The listing builds one solid part. Answer for the finished solid, in the listing's coordinates (mm). A direction names the side the tool comes from. Coordinates: 2 decimals unless noted, no trailing zeros. Order: outer loops, then holes, each group sorted by start corner. A loop starts at its lowest first (then second) coordinate and runs counter-clockwise, first axis right, second up.
```python
from build123d import *

# Parameters (mm, degrees)
SKETCH1_W           = 20
SKETCH1_H           = 18
BOSS_EXTRUDE1_DEPTH = 13
SKETCH7_W           = 3.5
SKETCH7_H           = 5.75
CUT_EXTRUDE6_DEPTH  = 25.351591324
SKETCH2_W           = 5.1
SKETCH2_H           = 11.1
CUT_EXTRUDE1_DEPTH  = 13.75
SKETCH3_R           = 1.05
CUT_EXTRUDE2_DEPTH  = 21.953818268
SKETCH4_R           = 2
CUT_EXTRUDE3_DEPTH  = 1.9
SKETCH11_R          = 0.9
CUT_EXTRUDE9_DEPTH  = 3
SKETCH5_W           = 11.1
SKETCH5_H           = 5.1
CUT_EXTRUDE4_DEPTH  = 19.708286934
SKETCH8_W           = 5.35
SKETCH8_H           = 5.1
SKETCH8_R           = 1.1
BOSS_EXTRUDE2_DEPTH = 1.5
SKETCH10_R          = 0.95
CUT_EXTRUDE8_DEPTH  = 6
SKETCH14_R          = 1.1
CUT_EXTRUDE11_DEPTH = 19.708286934
FILLET2_R           = 1.75
CHAMFER1_SIZE       = 0.5


with BuildPart() as part:
    # Sketch1 → Boss-Extrude1 (new body)
    with BuildSketch(Plane(origin=(0, 0, 0), x_dir=(1, 0, 0), z_dir=(0, 1, 0))):
        Rectangle(SKETCH1_W, SKETCH1_H)
    extrude(amount=BOSS_EXTRUDE1_DEPTH)

    # Sketch7 → Cut-Extrude6 (cut, through all)
    with BuildSketch(Plane.XY.offset(9)):
        with Locations((1, 10.125)):
            Rectangle(SKETCH7_W, SKETCH7_H)
    extrude(amount=-CUT_EXTRUDE6_DEPTH, mode=Mode.SUBTRACT)

    # Sketch2 → Cut-Extrude1 (cut)
    with BuildSketch(Plane.ZY.offset(10)):
        with Locations((-1.45, 7.45)):
            Rectangle(SKETCH2_W, SKETCH2_H)
    extrude(amount=-CUT_EXTRUDE1_DEPTH, mode=Mode.SUBTRACT)

    # Sketch3 → Cut-Extrude2 (cut, through all)
    with BuildSketch(Plane.ZY.offset(-3.75)):
        with Locations((-1.45, 3.9)):
            Circle(SKETCH3_R)
    extrude(amount=-CUT_EXTRUDE2_DEPTH, mode=Mode.SUBTRACT)

    # Sketch4 → Cut-Extrude3 (cut)
    with BuildSketch(Plane(origin=(10, 0, 0), x_dir=(0, 0, -1), z_dir=(1, 0, 0))):
        with Locations((1.45, 3.9)):
            Circle(SKETCH4_R)
    extrude(amount=-CUT_EXTRUDE3_DEPTH, mode=Mode.SUBTRACT)

    # Sketch11 → Cut-Extrude9 (cut)
    with BuildSketch(Plane(origin=(10, 0, 0), x_dir=(0, 0, -1), z_dir=(1, 0, 0))):
        with Locations((4.95, 3.9)):
            Circle(SKETCH11_R)
        with Locations(Location((-2.05, 3.9, 0), (0, 0, 180))):
            Circle(SKETCH11_R)
    extrude(amount=-CUT_EXTRUDE9_DEPTH, mode=Mode.SUBTRACT)

    # Sketch5 → Cut-Extrude4 (cut, through all)
    with BuildSketch(Plane(origin=(0, 13, 0), x_dir=(1, 0, 0), z_dir=(0, 1, 0))):
        with Locations((-0.55, -4.65)):
            Rectangle(SKETCH5_W, SKETCH5_H)
    extrude(amount=-CUT_EXTRUDE4_DEPTH, mode=Mode.SUBTRACT)

    # Sketch8 → Boss-Extrude2 (add)
    with BuildSketch(Plane(origin=(0, 13, 0), x_dir=(1, 0, 0), z_dir=(0, 1, 0))):
        with Locations((-3.425, -4.65)):
            Rectangle(SKETCH8_W, SKETCH8_H)
        with Locations(Location((-4.05, -4.65, 0), (0, 0, 270))):
            Circle(SKETCH8_R, mode=Mode.SUBTRACT)
    extrude(amount=-BOSS_EXTRUDE2_DEPTH)

    # Sketch10 → Cut-Extrude8 (cut)
    with BuildSketch(Plane(origin=(0, 13, 0), x_dir=(1, 0, 0), z_dir=(0, 1, 0))):
        with Locations(Location((-8.05, -6.825, 0), (0, 0, 270))):
            Circle(SKETCH10_R)
        with Locations(Location((7.5, 6.5, 0), (0, 0, 270))):
            Circle(SKETCH10_R)
    extrude(amount=-CUT_EXTRUDE8_DEPTH, mode=Mode.SUBTRACT)

    # Sketch14 → Cut-Extrude11 (cut, through all)
    with BuildSketch(Plane(origin=(0, 13, 0), x_dir=(1, 0, 0), z_dir=(0, 1, 0))):
        with Locations(Location((-7.5, 6.5, 0), (0, 0, 270))):
            Circle(SKETCH14_R)
        with Locations(Location((7.5, -6.5, 0), (0, 0, 270))):
            Circle(SKETCH14_R)
    extrude(amount=-CUT_EXTRUDE11_DEPTH, mode=Mode.SUBTRACT)

    # Fillet2
    fillet2_edges = [part.edges().sort_by_distance(p)[0] for p in [
        (2.75, 7.25, 8.1),
        (2.75, 7.25, 1.6),
        (-0.75, 7.25, 8.1),
        (-0.75, 7.25, 1.6),
        (2.75, 7.25, -6.5),
        (-0.75, 7.25, -6.5),
    ]]
    fillet(fillet2_edges, radius=FILLET2_R - 0.0001)  # a hair under: the kernel refuses the full size

    # Chamfer1
    chamfer1_edges = [part.edges().sort_by_distance(p)[0] for p in [
        (-0.55, 0, 2.1),
        (-0.55, 0, 7.2),
        (-6.1, 0, 4.65),
        (5, 0, 4.65),
    ]]
    chamfer(chamfer1_edges, length=CHAMFER1_SIZE)


solid = part.part
```
(1) Find section C-C (z = -1.45). Write down the section's boundary in (x, y).
(2) Find section B-B (x = 4.5). Write down the section's boundary in (y, z), and give its area (3 significant figures).
(3) Find section D-D (y = 9.25). Write down the section's boundary in (x, z) (3 decimals).
(4) Find section A-A (x = 7.5). Write down the section's boundary in (y, z).
(5) Each of these flat-tipped pins is pushed along its axis until it touches: pin 1 Ø4 at (x, z) = (1, 4.5) entering from -Y; pin 2 Ø1.8 at (x, z) = (7.5, 6.5) entering from -Y; pin 3 Ø1.5 at (x, z) = (-2, -1) entering from +Y. Where does it stop, or does it pass through?
(6) Consider line 1 (X direction, y = 11.65, z = -6.5); line 2 (Z direction, x = -3.25, y = 4); line 3 (Y direction, x = 7.2, z = -1.45). Determine where each line is inside the solid, lowest interval first.
(7) For faces 1 (the face through (8, 7, -7)), 2 (the face through (2.251, 7.776, -6.535)), 3 (the face through (-6.1, 6, 5)), determine the directions among +Z, -Z, +X, -X, +Y, -Y from which every point of the face is accessible in a straight line to the end or side of a thin tool.
(8) The mould has two halves that part along Z. Classify faces 4 (the face through (0, 6, -9)), 5 (the face through (-0.75, 12, 5)), 6 (the face through (8.14, 10.04, -7.2)): released by +Z, released by -Z, zero draft, split by the parting line, or undercut.
Findings below:
1. outline: (-10, 0) - (10, 0) - (10, 1.9) - (8.1, 1.9) - (8.1, 2.85) - (3.75, 2.85) - (3.75, 1.9) - (-10, 1.9) - close; (3.75, 4.95) - (8.1, 4.95) - (8.1, 5.9) - (10, 5.9) - (10, 13) - (3.75, 13) - close
2. outline: (0, -9) - (13, -9) - (13, 2.1) - (0.5, 2.1) - (0, 1.6) - close; (0, 7.7) - (0.5, 7.2) - (13, 7.2) - (13, 9) - (0, 9) - close; hole circle Ø2.1 at (3.9, -1.45)
2. area: 164 mm2
3. outline: (-10, -9) - (-0.75, -9) - (-0.75, -4) - (-10, -4) - close; (-10, 1.1) - (-0.75, 1.1) - (-0.75, 2.1) - (-6.1, 2.1) - (-6.1, 7.2) - (-0.75, 7.2) - (-0.75, 9) - (-10, 9) - close; (2.75, -9) - (10, -9) - (10, 9) - (2.75, 9) - (2.75, 7.2) - (5, 7.2) - (5, 2.1) - (2.75, 2.1) - (2.75, 1.1) - (3.75, 1.1) - (3.75, -4) - (2.75, -4) - close; hole circle Ø1.9 at (-8.05, 6.825); hole circle Ø2.2 at (-7.5, -6.5); hole circle Ø2.2 at (7.5, 6.5); hole circle Ø1.9 at (7.5, -6.5)
4. outline: (0, -9) - (13, -9) - (13, -7.45) - (7, -7.45) - (7, -5.55) - (13, -5.55) - (13, 5.4) - (0, 5.4) - close; (0, 7.6) - (13, 7.6) - (13, 9) - (0, 9) - close; hole circle Ø2.1 at (3.9, -1.45); hole circle Ø1.8 at (3.9, -4.95); hole circle Ø1.8 at (3.9, 2.05)
5. pin 1: stops at y = 11.5
5. pin 2: passes through
5. pin 3: stops at y = 1.9
6. line 1: x = -10 to -8.6, -6.4 to -0.75, 2.75 to 6.55, 8.45 to 10
6. line 2: z = -9 to -4, 1.1 to 2.1, 7.2 to 9
6. line 3: y = 0 to 2.85, 4.95 to 13
7. face 1: +Y
7. face 2: +Z, -Z, +Y
7. face 3: -Y
8. face 4: released by -Z
8. face 5: zero draft
8. face 6: undercut
